Can you work these out from the model? Positions are in its coordinate system, mm. Round coordinates to 2 decimals unless told otherwise and drop trailing zeros. Write each loop counter-clockwise with the first axis right and the second up, starting at its lowest first coordinate (ties: lowest second). Pieces come first, ordered by that corner, then holes. Notation, with made-up numbers: (64, 81.5) - (101, 81.5) arc R18 cw to (101, 106.5) - close; hole circle Ø1 at (66.5, -10). An arc over 180 degrees is marked (long way). One line per item, written item: value. Start each with the question number.
(1) I want a section at A-A on y = 154. List the corners of the cut face in (x, z) for me.
(2) I'm going to push flat-ended pins straight in: pin 1 Ø1.5 at (y, z) = (165, 2.5) entering from +X; pin 2 Ø3 at (y, z) = (229, 0.5) entering from -X; pin 3 Ø1.2 at (y, z) = (-228, -0.5) entering from +X. Where does each tip first touch, or does it pass through?
(3) If I drill on L1, parallel to Z at x = 1, y = -209; L2, parallel to X at y = 14, z = 0.25, over which ranges is the centre line in solid material (lowest first)? Write a range as from..to.
from build123d import *

# Parameters (mm, degrees)
SKETCH1_R                = 3.3
BOSS_EXTRUDE1_DEPTH      = 245
BOSS_EXTRUDE1_DEPTH_BACK = 245
SKETCH2_OUTSIDE_W        = 106.618
SKETCH2_OUTSIDE_H        = 106.618
SKETCH2_OUTSIDE_W_2      = 5.3
SKETCH2_OUTSIDE_H_2      = 5.3
CUT_EXTRUDE1_DEPTH       = 60
SKETCH3_OUTSIDE_W        = 107.928
SKETCH3_OUTSIDE_H        = 107.928
CUT_EXTRUDE2_DEPTH       = 15
CUT_EXTRUDE2_TAPER       = 2.5
SKETCH4_OUTSIDE_W        = 106.618
SKETCH4_OUTSIDE_H        = 106.618
SKETCH4_OUTSIDE_W_2      = 5.3
SKETCH4_OUTSIDE_H_2      = 5.3
CUT_EXTRUDE3_DEPTH       = 60
SKETCH5_OUTSIDE_W        = 107.928
SKETCH5_OUTSIDE_H        = 107.928
CUT_EXTRUDE4_DEPTH       = 15
CUT_EXTRUDE4_TAPER       = 2.5


with BuildPart() as part:
    # Sketch1 → Boss-Extrude1 (new body, two sides)
    with BuildSketch(Plane(origin=(0, 0, 0), x_dir=(1, 0, 0), z_dir=(0, 1, 0))) as boss_extrude1_sk:
        Circle(SKETCH1_R)
    extrude(amount=BOSS_EXTRUDE1_DEPTH)
    extrude(boss_extrude1_sk.sketch, amount=-BOSS_EXTRUDE1_DEPTH_BACK)

    # Sketch2 outside → Cut-Extrude1 (cut)
    with BuildSketch(Plane(origin=(0, 245, 0), x_dir=(1, 0, 0), z_dir=(0, 1, 0))):
        Rectangle(SKETCH2_OUTSIDE_W, SKETCH2_OUTSIDE_H)
        Rectangle(SKETCH2_OUTSIDE_W_2, SKETCH2_OUTSIDE_H_2, mode=Mode.SUBTRACT)
    extrude(amount=-CUT_EXTRUDE1_DEPTH, mode=Mode.SUBTRACT)

    # Sketch3 outside → Cut-Extrude2 (cut)
    with BuildSketch(Plane(origin=(0, 185, 0), x_dir=(1, 0, 0), z_dir=(0, 1, 0))):
        Rectangle(SKETCH3_OUTSIDE_W, SKETCH3_OUTSIDE_H)
        Polygon((-1.966596044, -2.65), (1.966596044, -2.65), (2.65, -2.65), (2.65, -1.966596044), (2.65, 1.966596044), (2.65, 2.65), (1.966596044, 2.65), (-1.966596044, 2.65), (-2.65, 2.65), (-2.65, 1.966596044), (-2.65, -1.966596044), (-2.65, -2.65), align=None, mode=Mode.SUBTRACT)
    extrude(amount=-CUT_EXTRUDE2_DEPTH, taper=CUT_EXTRUDE2_TAPER, mode=Mode.SUBTRACT)

    # Sketch4 outside → Cut-Extrude3 (cut)
    with BuildSketch(Plane.XZ.offset(245)):
        Rectangle(SKETCH4_OUTSIDE_W, SKETCH4_OUTSIDE_H)
        Rectangle(SKETCH4_OUTSIDE_W_2, SKETCH4_OUTSIDE_H_2, mode=Mode.SUBTRACT)
    extrude(amount=-CUT_EXTRUDE3_DEPTH, mode=Mode.SUBTRACT)

    # Sketch5 outside → Cut-Extrude4 (cut)
    with BuildSketch(Plane.XZ.offset(185)):
        Rectangle(SKETCH5_OUTSIDE_W, SKETCH5_OUTSIDE_H)
        Polygon((1.966596044, -2.65), (2.65, -2.65), (2.65, -1.966596044), (2.65, 1.966596044), (2.65, 2.65), (1.966596044, 2.65), (-1.966596044, 2.65), (-2.65, 2.65), (-2.65, 1.966596044), (-2.65, -1.966596044), (-2.65, -2.65), (-1.966596044, -2.65), align=None, mode=Mode.SUBTRACT)
    extrude(amount=-CUT_EXTRUDE4_DEPTH, taper=CUT_EXTRUDE4_TAPER, mode=Mode.SUBTRACT)


solid = part.part
Established:
1. outline: circle Ø6.6 at (0, 0)
2. pin 1: x = 2.8
2. pin 2: x = -2.65
2. pin 3: x = 2.65
3. L1: -2.65..2.65
3. L2: -3.29..3.29
